Design review of the part built by this model. Coordinates are the model's own, in mm. Face numbers are marked on the shaded views. Round coordinates to 2 decimals unless told otherwise and drop trailing zeros. Loops run counter-clockwise (first coordinate to the right, second up) from the corner with the lowest first, then second, coordinate; pieces in that order, holes last. Notation, with made-up numbers: (44.5, -11.75) - (96.5, -11.75) arc R21 cw to (96.5, -4.75) - close; hole circle Ø1 at (14, -21). An arc over 180 degrees is marked (long way). Return JSON: item names as keys, results as strings. Group by question number.
(1) We need section C-C, the plane y = 8.5. Write out the cut boundary in (x, z).
(2) We need section D-D, the plane z = -0.7. Write out the cut boundary in (x, y), and give its area (3 significant figures).
(3) Clearance check with a flat-ended pin moving along its axis: pin 1 (1 mm diameter, centred on y = 6, z = 0.5, fed in from -X). State where the tip first meets the part, or that it passes through.
(4) Wall thickness on L1, parallel to Y at x = 0.35, z = 0.05; L2, parallel to X at y = 5.75, z = 0; L3, parallel to Z at x = -0.05, y = 5: over which ranges is each line inside the solid? List them lowest first. Write a range as [from, to].
(5) We need section B-B, the plane z = 0. Write out the cut boundary in (x, y), and give its area (3 significant figures).
(6) We need section A-A, the plane x = 0. Write out the cut boundary in (y, z), and give its area (3 significant figures).
(7) The part is to be moulded in two halves that separate along Y. For the marked faces 1, 2, 3 and 4, say which applies: pulls with the +Y half, pulls with the -Y half, needs draft (parallel to the pull), parting line crosses it, or undercut.
Autodesk Inventor part; units mm, degrees
ref_plane "РабПлоскость1" through (0, 0, 0) normal (-1, 0, 0) x (0, 0, 1)
ref_plane "YZ Plane" through (0, 0, 0) normal (1, 0, 0) x (0, 1, 0)
ref_plane "XZ Plane" through (0, 0, 0) normal (0, 1, 0) x (-1, 0, 0)
sketch "Эскиз1" plane through (0, 0, 0) normal (0, 1, 0) x (-1, 0, 0)
  circle A0 centre (0, 0) radius 0.5
  dimension "d0" = 1
extrude "Выдавливание1" add sketch "Эскиз1" along normal blind 12
sketch "Эскиз2" plane through (0, 0, 0) normal (1, 0, 0) x (0, 1, 0)
  line L0 (0, 0) -> (6, 0) construction
  circle A0 centre (6, 0) radius 1
  dimension "d3" = 6
  dimension "d4" = 2
extrude "Выдавливание2" add sketch "Эскиз2" along normal mid plane 0.5
sketch "Эскиз3" plane through (-0.25, 0, 0) normal (-1, 0, 0) x (0, 0, 1)
  line L0 (0, 0) -> (0, 6) construction
  circle A0 centre (0, 6) radius 1
  dimension "d7" = 6
  dimension "d8" = 2
extrude "Выдавливание3" cut sketch "Эскиз3" along normal blind 1.25
sketch "Эскиз4" plane through (-0.25, 0, 0) normal (-1, 0, 0) x (0, 0, 1)
  point P0 (0, 0)
ref_plane "РабПлоскость1" through (0, 0, 0) normal (-1, 0, 0) x (0, 0, 1)
sketch "Эскиз6" plane through (0.25, 0, 0) normal (1, 0, 0) x (0, 0, -1)
  circle A0 centre (0, 6) radius 1
  point P0 (0, 0)
extrude "Выдавливание5" cut sketch "Эскиз6" along normal blind 3
properties part number "штырь"
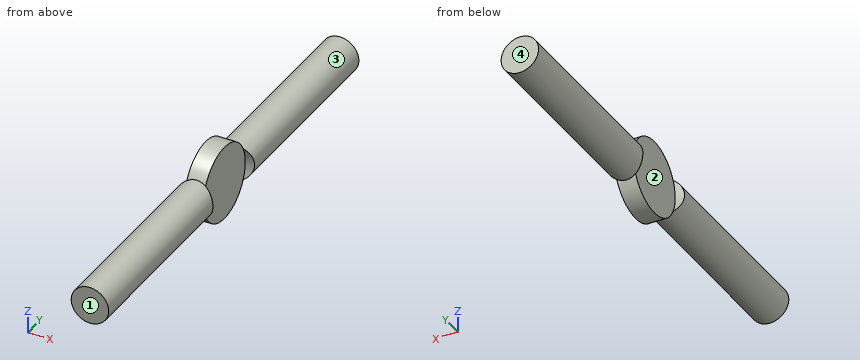
Solutions:
{
 "1": {"outline": "circle Ø1 at (0, 0)"},
 "2": {"outline": "(-0.25, 5.29) - (0.25, 5.29) - (0.25, 6.71) - (-0.25, 6.71) - close", "area": "0.714 mm^2"},
 "3": {"pin 1": "x = -0.25"},
 "4": {"L1": "[0, 5], [7, 12]", "L2": "[-0.25, 0.25]", "L3": "[-0.5, 0.5]"},
 "5": {"outline": "(-0.5, 0) - (0.5, 0) - (0.5, 5) - (0.25, 5) - (0.25, 7) - (0.5, 7) - (0.5, 12) - (-0.5, 12) - (-0.5, 7) - (-0.25, 7) - (-0.25, 5) - (-0.5, 5) - close", "area": "11.0 mm^2"},
 "6": {"outline": "(0, -0.5) - (5.13, -0.5) arc R1 ccw to (6.87, -0.5) - (12, -0.5) - (12, 0.5) - (6.87, 0.5) arc R1 ccw to (5.13, 0.5) - (0, 0.5) - close", "area": "13.2 mm^2"},
 "7": {"face 1": "pulls with the -Y half", "face 2": "undercut", "face 3": "needs draft", "face 4": "pulls with the +Y half"}
}
